from build123d import *

# Parameters (mm, degrees)
F0_W           = 46
F0_H           = 36
F0_R           = 10
F1_DEPTH       = 10
F3_D           = 5.5
F3_DEPTH       = 9
F3_CBORE_D     = 9.75
F3_CBORE_DEPTH = 5
F3_TIP         = 1.6523667023
F4_R           = 10
F5_DEPTH       = 6


with BuildPart() as f1:
    # F0 (on Front) → F1 (new body)
    with BuildSketch(Plane.XZ):
        Rectangle(F0_W, F0_H)
        with Locations((-7, 3)):
            Circle(F0_R, mode=Mode.SUBTRACT)
    extrude(amount=F1_DEPTH)

    # F3
    with Locations(Plane(origin=(0, 0, 0), x_dir=(-1, 0, 0), z_dir=(0, 1, 0))):
        with Locations((-17.0919913413, 12), (-16.9995214964, -6)):
            CounterBoreHole(F3_D / 2, F3_CBORE_D / 2, F3_CBORE_DEPTH, depth=F3_DEPTH)
            with Locations((0, 0, -(F3_DEPTH + F3_TIP / 2))):  # 118° drill point
                Cone(0, F3_D / 2, F3_TIP, mode=Mode.SUBTRACT)

    # F4 (on face) → F5 (cut)
    with BuildSketch(Plane(origin=(0, 0, 0), x_dir=(-1, 0, 0), z_dir=(0, 1, 0))):
        with BuildLine():
            Line((-7.9965220779, 18), (-7.9965220779, 3.3229946864))
            Line((-7.9965220779, 3.3229946864), (-7.9965220779, 2.6770053136))
            ThreePointArc((-7.9965220779, 2.6770053136), (-3.0413947673, -8.1431768867), (8.2344393019, -11.9491190245))
            Line((8.2344393019, -11.9491190245), (23, -11.9491190245))
            Line((23, -11.9491190245), (23, 18))
            Line((23, 18), (-7.9965220779, 18))
        make_face()
        with Locations((7, 3)):
            Circle(F4_R, mode=Mode.SUBTRACT)
    extrude(amount=-F5_DEPTH, mode=Mode.SUBTRACT)


solid = f1.part
Design review of the part built by this model. Coordinates are the model's own, in mm. A direction names the side the tool comes from. Give positions to 0.01 mm unless a question says otherwise; leave off trailing zeros. Order: outer loops, then holes, each group sorted by start corner. A loop starts at its lowest first (then second) coordinate and runs counter-clockwise, first axis right, second up. Notation, with made-up numbers: (-13, -38.75) - (29, -38.75) arc R23 cw to (29, -15.75) - close; hole circle Ø9 at (50, 39). An arc over 180 degrees is marked (long way). Write item = value, one per line. Start each with the question number.
Q1. Mouldability with a two-part tool opening along X and no side actions: class faces 1 (the face through (-16, -3, -11.949)), 2 (the face through (19.54, -7.03, -7.05)), 3 (the face through (23, -5, 0)) as released by +X, released by -X, zero draft, split by the parting line, or undercut.
Q2. We need section D-D on y = -1.5. State the section outline as (x, z) points (3 decimals), plus the area to 3 significant figures.
Q3. We need section C-C on z = -6. State the section outline as (x, y) points.
Q4. Tool access review of faces 4 (the face through (0, -5, -18)), 5 (the face through (7.997, -3, 10)), 6 (the face through (15, -5, 9.9)): name each direction out of +Z, -Z, +X, -X, +Y, -Y from which nothing blocks a thin tool from reaching the whole face with its end or side.
Q5. To check wall thickness, follow L1, parallel to X at y = -6.75, z = -4; L2, parallel to Y at x = -3, z = 13; L3, parallel to X at y = -8, z = -6. State the ranges of each line that lie inside material, in increasing order. Write a range as from..to.
Q6. Clearance check with flat-ended pins moving along their axes: pin 1 Ø3 at (x, y) = (-15, -2) entering from +Z; pin 2 Ø3 at (x, z) = (18, -5) entering from +Y; pin 3 Ø1.8 at (y, z) = (-4, 12) entering from -X. State where each tip first meets the part, or that it passes through.
Q7. We need section B-B on y = -6.75. State the section outline as (x, z) points.
Q8. We need section A-A on x = -15. State the section outline as (y, z) points.
Working result:
q1.face_1 = zero draft
q1.face_2 = undercut
q1.face_3 = released by +X
q2.outline = (-23, -18) - (23, -18) - (23, 18) - (7.997, 18) - (7.997, 2.677) arc R15 cw to (-8.234, -11.949) - (-23, -11.949) - close; hole circle Ø9.75 at (17, -6); hole circle Ø9.75 at (17.092, 12)
q2.area = 626 mm²
q3.outline = (-23, -10) - (-11.36, -10) - (-11.36, -6) - (-23, -6) - close; (-2.64, -10) - (15.91, -10) - (14.25, -9) - (14.25, -5) - (12.12, -5) - (12.12, 0) - (5, 0) - (5, -6) - (-2.64, -6) - close; (18.09, -10) - (23, -10) - (23, 0) - (21.87, 0) - (21.87, -5) - (19.75, -5) - (19.75, -9) - close
q4.face_4 = -Z, +X, -X, +Y, -Y
q4.face_5 = +Z, -X, +Y
q4.face_6 = +Y
q5.L1 = -23..-14.14, 0.14..15.11, 18.89..23
q5.L2 = -10..-6
q5.L3 = -23..-11.36, -2.64..14.25, 19.75..23
q6.pin_1 = -11.95
q6.pin_2 = -5
q6.pin_3 = 8
q7.outline = (-23, -18) - (23, -18) - (23, 18) - (-23, 18) - close; hole circle Ø20 at (-7, 3); hole circle Ø5.5 at (17, -6); hole circle Ø5.5 at (17.09, 12)
q8.outline = (-10, -18) - (0, -18) - (0, -11.95) - (-6, -11.95) - (-6, -3) - (-10, -3) - close; (-10, 9) - (-6, 9) - (-6, 18) - (-10, 18) - close
